Build history of the part. All positions in model axes, mm. A direction names the side the tool comes from. Round coordinates to 2 decimals unless told otherwise and drop trailing zeros. Loops run counter-clockwise (first coordinate to the right, second up) from the corner with the lowest first, then second, coordinate; pieces in that order, holes last.
from build123d import *

# Parameters (mm, degrees)
SKETCH2_W           = 70
SKETCH2_H           = 30
SKETCH2_R           = 1.25
BOSS_EXTRUDE1_DEPTH = 4
SKETCH4_W           = 30
SKETCH4_H           = 20
BOSS_EXTRUDE2_DEPTH = 60.0001011
SKETCH5_W           = 70
SKETCH5_H           = 30
SKETCH5_R           = 2.7
BOSS_EXTRUDE3_DEPTH = 4


with BuildPart() as part:
    # Sketch2 → Boss-Extrude1 (new body)
    with BuildSketch(Plane(origin=(0, 0, 0), x_dir=(1, 0, 0), z_dir=(0, 1, 0))):
        Rectangle(SKETCH2_W, SKETCH2_H)
        with Locations((-30, -12.5)):
            Circle(SKETCH2_R, mode=Mode.SUBTRACT)
        with Locations((-30, 12.5)):
            Circle(SKETCH2_R, mode=Mode.SUBTRACT)
        with Locations((30, -12.5)):
            Circle(SKETCH2_R, mode=Mode.SUBTRACT)
        with Locations((30, 12.5)):
            Circle(SKETCH2_R, mode=Mode.SUBTRACT)
    extrude(amount=BOSS_EXTRUDE1_DEPTH)

    # Sketch4 → Boss-Extrude2 (add)
    with BuildSketch(Plane(origin=(0, 4, 0), x_dir=(1, 0, 0), z_dir=(0, 1, 0))):
        Rectangle(SKETCH4_W, SKETCH4_H)
    extrude(amount=BOSS_EXTRUDE2_DEPTH)

    # Sketch5 → Boss-Extrude3 (add)
    with BuildSketch(Plane(origin=(0, 64.0001011, 0), x_dir=(1, 0, 0), z_dir=(0, 1, 0))):
        Rectangle(SKETCH5_W, SKETCH5_H)
        with Locations((-28, 0)):
            Circle(SKETCH5_R, mode=Mode.SUBTRACT)
        with Locations((28, 0)):
            Circle(SKETCH5_R, mode=Mode.SUBTRACT)
    extrude(amount=BOSS_EXTRUDE3_DEPTH)


solid = part.part
(1) Slice it at D-D on z = 8.5. List the corners of the cut face in (x, y), plus the area to 3 significant figures.
Responses:
outline: (-35, 0) - (35, 0) - (35, 4) - (15, 4) - (15, 64) - (35, 64) - (35, 68) - (-35, 68) - (-35, 64) - (-15, 64) - (-15, 4) - (-35, 4) - close
area: 2,360 mm2
(2) Slice it at B-B on z = 12.5. List the corners of the cut face in (x, y).
Responses:
outline: (-35, 0) - (-31.25, 0) - (-31.25, 4) - (-35, 4) - close; (-35, 64) - (35, 64) - (35, 68) - (-35, 68) - close; (-28.75, 0) - (28.75, 0) - (28.75, 4) - (-28.75, 4) - close; (31.25, 0) - (35, 0) - (35, 4) - (31.25, 4) - close
(3) Slice it at A-A on x = -16. List the corners of the cut face in (y, z), plus the area to 3 significant figures.
Responses:
outline: (0, -15) - (4, -15) - (4, 15) - (0, 15) - close; (64, -15) - (68, -15) - (68, 15) - (64, 15) - close
area: 240 mm2
(4) Pin check, flat tips, straight feed: P1, Ø8, axis at x = 6.5, y = 32, coming from the +Z side; P2, Ø10, axis at y = 47.5, z = 2, coming from the -X side; P3, Ø10, axis at y = 31, z = 10.5, coming from the +X side. Stop position of each tip, or through.
Responses:
P1: stops at z = 10
P2: stops at x = -15
P3: stops at x = 15
(5) Which spindle directions (+Z, -Z, +X, -X, +Y, -Y) get a long thin tool onto all of the face, cutting with end or side? Do faces 1 (the face through (30.672, 1.972, -13.554)), 2 (the face through (0, 34, -10)), 3 (the face through (0, 34, 10)). Say none if no direction does.
Responses:
face 1: -Y
face 2: -Z, +X, -X
face 3: +Z, +X, -X
(6) Slice it at C-C on x = -4. List the corners of the cut face in (y, z), plus the area to 3 significant figures.
Responses:
outline: (0, -15) - (4, -15) - (4, -10) - (64, -10) - (64, -15) - (68, -15) - (68, 15) - (64, 15) - (64, 10) - (4, 10) - (4, 15) - (0, 15) - close
area: 1,440 mm2
(7) Pull direction X, two halves, no side cores. Call faces 4 (the face through (-29.328, 1.972, 11.446)), 5 (the face through (35, 66, 0)), 6 (the face through (-0.5, 64, -10.2)): +X half, -X half, draft (parallel to the pull), parting line (faces both ways), or undercut.
Responses:
face 4: undercut
face 5: +X half
face 6: draft
(8) Probe line 1 (Z direction, x = -30, y = 2.3); line 2 (X direction, y = 1.05, z = 12.5); line 3 (Y direction, x = 24, z = 11.5). List the from-to ranges inside material, lowest first.
Responses:
line 1: z = -15 to -13.75, -11.25 to 11.25, 13.75 to 15
line 2: x = -35 to -31.25, -28.75 to 28.75, 31.25 to 35
line 3: y = 0 to 4, 64 to 68
